Read the model definition and answer for the solid it produces. Units are mm, in the model's axes. A direction names the side the tool comes from. Round coordinates to 2 decimals unless told otherwise and drop trailing zeros. Order: outer loops, then holes, each group sorted by start corner. A loop starts at its lowest first (then second) coordinate and runs counter-clockwise, first axis right, second up.
from build123d import *

# Parameters (mm, degrees)
SKETCH_2_W      = 515
SKETCH_2_H      = 360
EXTRUDE_1_DEPTH = 285
SKETCH_3_R      = 12
EXTRUDE_2_DEPTH = 20
SKETCH_4_W      = 36.17518645
SKETCH_4_H      = 191.327135514
EXTRUDE_3_DEPTH = 25
SKETCH_5_W      = 388.964610797
SKETCH_5_H      = 188.668975617
EXTRUDE_4_DEPTH = 85
EXTRUDE_4_TAPER = 18


with BuildPart() as part:
    # Эскиз2 → Бобышка-Вытянуть1 (new body)
    with BuildSketch(Plane(origin=(0, 0, 0), x_dir=(1, 0, 0), z_dir=(0, 1, 0))):
        with Locations((257.5, 180)):
            Rectangle(SKETCH_2_W, SKETCH_2_H)
    extrude(amount=EXTRUDE_1_DEPTH)

    # Эскиз3 → Бобышка-Вытянуть2 (add)
    with BuildSketch(Plane.XZ):
        with Locations((30, -25)):
            Circle(SKETCH_3_R)
        with Locations((30, -335)):
            Circle(SKETCH_3_R)
        with Locations((485, -335)):
            Circle(SKETCH_3_R)
        with Locations((485, -25)):
            Circle(SKETCH_3_R)
    extrude(amount=EXTRUDE_2_DEPTH)

    # Эскиз4 → Бобышка-Вытянуть3 (add)
    with BuildSketch(Plane.XY):
        with Locations((400.600187064, 145.73424428)):
            Rectangle(SKETCH_4_W, SKETCH_4_H)
    extrude(amount=EXTRUDE_3_DEPTH)

    # Эскиз5 → Бобышка-Вытянуть4 (add)
    with BuildSketch(Plane(origin=(0, 0, -360), x_dir=(-1, 0, 0), z_dir=(0, 0, -1))):
        with Locations((-254.857577373, 150.431495615)):
            Rectangle(SKETCH_5_W, SKETCH_5_H)
    extrude(amount=EXTRUDE_4_DEPTH, taper=EXTRUDE_4_TAPER)


solid = part.part
Q1. A cutting plane is placed at B-B, the plane x = 485. Give the vertices of the cut face in (y, z), plus the area to 3 significant figures.
Outcome:
outline: (-20, -347) - (0, -347) - (0, -360) - (285, -360) - (285, 0) - (0, 0) - (0, -13) - (-20, -13) - (-20, -37) - (0, -37) - (0, -323) - (-20, -323) - close
area: 104,000 mm2
Q2. For faces 1 (the face through (41.446, -9.86, -21.396)), 2 (the face through (400, 241.398, 12)), 3 (the face through (382.513, 144, 12)), 4 (the face through (254, 46, -360)), 5 (the face through (400, 50.071, 12)), determine the directions among +Z, -Z, +X, -X, +Y, -Y from which every point of the face is accessible in a straight line to the end or side of a thin tool.
Outcome:
face 1: -Y
face 2: +Z, +X, -X, +Y
face 3: +Z, -X, +Y, -Y
face 4: -Z
face 5: +Z, +X, -X, -Y
Q3. A cutting plane is placed at A-A, the plane z = -335. Give the vertices of the cut face in (x, y), plus the area to 3 significant figures.
Outcome:
outline: (0, 0) - (18, 0) - (18, -20) - (42, -20) - (42, 0) - (473, 0) - (473, -20) - (497, -20) - (497, 0) - (515, 0) - (515, 285) - (0, 285) - close
area: 148,000 mm2
Q4. For a pull along X with two mould halves and no side action, classify faces 6 (the face through (496.085, -9.86, -339.596)), 7 (the face through (418.688, 144, 12)), 8 (the face through (496.446, -9.86, -21.396)), 9 (the face through (30, -20, -25)) as released by +X, released by -X, zero draft, split by the parting line, or undercut.
Outcome:
face 6: undercut
face 7: released by +X
face 8: undercut
face 9: zero draft
Q5. Straight lines are drawn through the part: probe 1 along Z at (x, y) = (83, 261); probe 2 along Z at (x, y) = (324.5, 196); probe 3 along Y at (x, z) = (386, -249). For each, find the intervals that lie inside material, in ascending order.
Outcome:
probe 1: z = -360 to 0
probe 2: z = -445 to 0
probe 3: y = 0 to 285
Q6. A cutting plane is placed at C-C, the plane z = -197.5. Give the vertices of the cut face in (x, y), plus the area to 3 significant figures.
Outcome:
outline: (0, 0) - (515, 0) - (515, 285) - (0, 285) - close
area: 147,000 mm2
Q7. Flat-ended cylindrical pins translate along their axes: pin 1 (1 mm diameter, centred on x = 331.5, y = 96.5, fed in from +Z); pin 2 (7.5 mm diameter, centred on x = 407.5, z = 8.5, fed in from +Y); pin 3 (6 mm diameter, centred on x = 313.5, y = 24.5, fed in from -Z); pin 4 (4 mm diameter, centred on y = 77.5, z = -204.5, fed in from -X). Find the tip coordinate at first contact, or state that the pin passes through.
Outcome:
pin 1: stops at z = 0
pin 2: stops at y = 241.4
pin 3: stops at z = -360
pin 4: stops at x = 0
